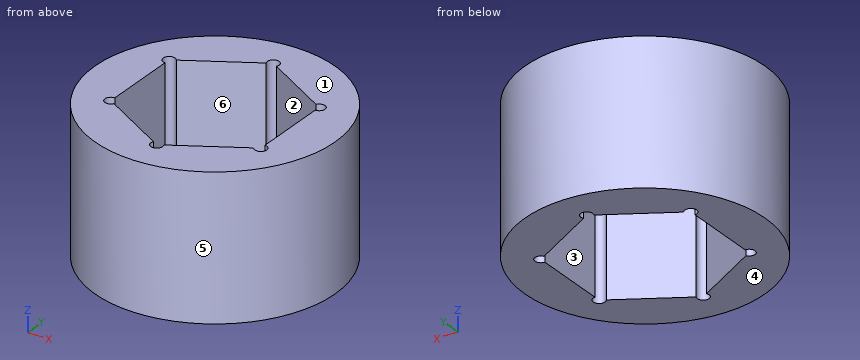
from build123d import *

# Parameters (mm, degrees)
F0_R     = 8
F1_DEPTH = 9.525


# Not quite as in the source:
# - a length typed as a fraction of an inch, garbled in the dataset ("3 / 203.2 mm" for 3/8 in), is restored


with BuildPart() as f1:
    # F0 (on Top) → F1 (new body)
    with BuildSketch(Plane.XY):
        Circle(F0_R)
        with BuildLine():
            ThreePointArc((-0.3437038321, 5.5750625), (0, 6.170375), (0.3437038321, 5.5750625))
            Line((0.3437038321, 5.5750625), (4.6562938366, 3.0851875))
            ThreePointArc((4.6562938366, 3.0851875), (5.3437015009, 3.0851875), (4.9999976687, 2.489875))
            Line((4.9999976687, 2.489875), (4.9999976687, -2.489875))
            ThreePointArc((4.9999976687, -2.489875), (5.3437015009, -3.0851875), (4.6562938366, -3.0851875))
            Line((4.6562938366, -3.0851875), (0.3437038321, -5.5750625))
            ThreePointArc((0.3437038321, -5.5750625), (0, -6.170375), (-0.3437038321, -5.5750625))
            Line((-0.3437038321, -5.5750625), (-4.6562938366, -3.0851875))
            ThreePointArc((-4.6562938366, -3.0851875), (-5.3437015009, -3.0851875), (-4.9999976687, -2.489875))
            Line((-4.9999976687, -2.489875), (-4.9999976687, 2.489875))
            ThreePointArc((-4.9999976687, 2.489875), (-5.3437015009, 3.0851875), (-4.6562938366, 3.0851875))
            Line((-4.6562938366, 3.0851875), (-0.3437038321, 5.5750625))
        make_face(mode=Mode.SUBTRACT)
    extrude(amount=F1_DEPTH)


solid = f1.part
Part model, mm, in its own coordinate system. Face numbers are marked on the shaded views. A direction names the side the tool comes from. Coordinates: 2 decimals unless noted, no trailing zeros. Order: outer loops, then holes, each group sorted by start corner. A loop starts at its lowest first (then second) coordinate and runs counter-clockwise, first axis right, second up. Notation, with made-up numbers: M -1,60 L 45,60 A23 cw 45,72 Z; hole C 38,19.25 d2. An arc over 180 degrees is marked long. One line per question, with ' | ' between items.
Q1. Drill centre lines: line 1 (X direction, y = 2, z = 7.25); line 2 (X direction, y = 0.25, z = 3.25); line 3 (Y direction, x = -3.5, z = 4.25). Where is each one in solid material? Low to high.
A:
line 1: x = -7.75 to -5, 5 to 7.75 | line 2: x = -8 to -5, 5 to 8 | line 3: y = -7.19 to -3.75, 3.75 to 7.19
Q2. Slice it at A-A (x = 0). Give the cut face in (y, z) (3 decimals).
A:
outline: M -8,0 L -6.17,0 L -6.17,9.525 L -8,9.525 Z; M 6.17,0 L 8,0 L 8,9.525 L 6.17,9.525 Z
Q3. 3-axis set-ups, long thin cutter, end or side, ignore diameter. For the marked faces 1 and 2: which of +Z, -Z, +X, -X, +Y, -Y reach the whole face in a straight line?
A:
face 1: +Z, +X, -X, +Y, -Y | face 2: +Z, -Z
Q4. Slice it at B-B (y = 0). Give the cut face in (x, z) (3 decimals).
A:
outline: M -8,0 L -5,0 L -5,9.525 L -8,9.525 Z; M 5,0 L 8,0 L 8,9.525 L 5,9.525 Z
Q5. Two-plate mould, pull along Y, no slides. Class the marked faces 3, 4, 5 and 6: +Y half, -Y half, draft (parallel to the pull), parting line (faces both ways), or undercut.
A:
face 3: undercut | face 4: draft | face 5: parting line | face 6: undercut
Q6. Slice it at C-C (z = 7.75). Give the cut face in (x, y).
A:
outline: C 0,0 d16; hole M -5,-2.49 A0.4 ccw long -4.66,-3.09 L -0.34,-5.58 A0.4 ccw long 0.34,-5.58 L 4.66,-3.09 A0.4 ccw long 5,-2.49 L 5,2.49 A0.4 ccw long 4.66,3.09 L 0.34,5.58 A0.4 ccw long -0.34,5.58 L -4.66,3.09 A0.4 ccw long -5,2.49 Z
Q7. Pin check, flat tips, straight feed: P1, Ø4, axis at x = 6, z = 8, coming from the -Y side; P2, Ø1.5, axis at y = 2, z = 3, coming from the -X side; P3, Ø2, axis at x = 3.5, z = 5, coming from the +Y side. Stop position of each tip, or through.
A:
P1: stops at y = -6.93 | P2: stops at x = -7.9 | P3: stops at y = 7.6
